Can you work these out from the model? Positions are in its coordinate system, mm. Face numbers are marked on the shaded views. A direction names the side the tool comes from. Round coordinates to 2 decimals unless told otherwise and drop trailing zeros. Write each loop counter-clockwise with the first axis right and the second up, starting at its lowest first coordinate (ties: lowest second). Pieces come first, ordered by that corner, then holes. Notation, with made-up numbers: M 20.5,9 L 41.5,9 A8 cw 41.5,22 Z; hole C 36.25,7.5 d11. An arc over 180 degrees is marked long. Answer as a JSON object with one key per item and string values. Group by question number.
1) Suppose I cut it at D-D, the plane y = 72. Write out the boundary of the cut face in (x, z).
2) Suppose I cut it at C-C, the plane z = -6.75. Write out the boundary of the cut face in (x, y), and give its area (3 significant figures).
3) I'm going to push flat-ended pins straight in: pin 1 Ø0.9 at (x, z) = (-24, -9) entering from +Y; pin 2 Ø1 at (x, z) = (-26, -3.5) entering from -Y; pin 3 Ø2 at (x, y) = (12.5, 17.5) entering from -Z; pin 4 Ø3 at (y, z) = (13.5, -6) entering from +X. Where does each tip first touch, or does it pass through?
4) Suppose I cut it at B-B, the plane x = -2.5. Write out the boundary of the cut face in (y, z).
5) Please list where these lines run through material, in increasing order: L1, parallel to Y at x = 0, z = -1.65; L2, parallel to Z at x = 11.5, y = 18.5; L3, parallel to Y at x = -23, z = 0.25. Write a range as [from, to].
6) On a 3-axis mill with a long thin cutter (end or side, diameter ignored), from which of +Z, -Z, +X, -X, +Y, -Y can I reach the whole of each face in a straight line? I mean the marked faces 4, 5 and 6. Say none if no direction works.
7) If we mould it in two halves opening along Y, with no side actions, what happens to the marked faces 1, 2 and 3? For each: +Y half, -Y half, draft (parallel to the pull), parting line (faces both ways), or undercut.
8) Suppose I cut it at A-A, the plane y = 29.5. Write out the boundary of the cut face in (x, z), and give its area (3 significant figures).
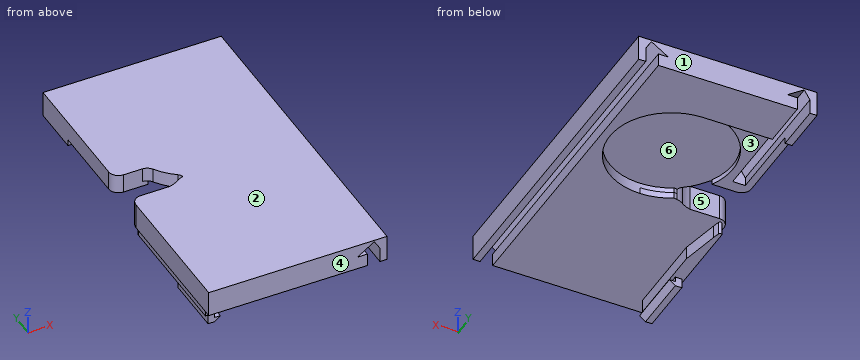
from build123d import *
from build123d.topology import SkipClean

# Parameters (mm, degrees)
SKETCH1_W           = 55
SKETCH1_H           = 8
BOSS_EXTRUDE1_DEPTH = 100
SKETCH4_R           = 19
CUT_EXTRUDE3_DEPTH  = 3.56
CUT_EXTRUDE4_DEPTH  = 2
CUT_EXTRUDE5_DEPTH  = 16
BOSS_EXTRUDE2_START = 2
BOSS_EXTRUDE2_DEPTH = 2
FILLET1_R           = 3
FILLET2_R           = 3
FILLET3_R           = 3
FILLET4_R           = 2
BOSS_EXTRUDE3_DEPTH = 4
CUT_EXTRUDE9_DEPTH  = 39
CUT_EXTRUDE13_DEPTH = 108
BOSS_EXTRUDE4_DEPTH = 18
FILLET5_R           = 0.5


with BuildPart() as part:
    # Sketch1 → Boss-Extrude1 (new body)
    with BuildSketch(Plane(origin=(0, 0, 0), x_dir=(1, 0, 0), z_dir=(0, 1, 0))):
        Rectangle(SKETCH1_W, SKETCH1_H)
    extrude(amount=BOSS_EXTRUDE1_DEPTH)

    # Sketch4 → Cut-Extrude3 (cut)
    with BuildSketch(Plane(origin=(0, 0, -4), x_dir=(-1, 0, 0), z_dir=(0, 0, -1))):
        with Locations((0, 65.948341349)):
            Circle(SKETCH4_R)
    extrude(amount=-CUT_EXTRUDE3_DEPTH, mode=Mode.SUBTRACT)

    # Sketch5 → Cut-Extrude4 (cut)
    with BuildSketch(Plane(origin=(0, 0, -4), x_dir=(-1, 0, 0), z_dir=(0, 0, -1))):
        with BuildLine():
            Line((0, 46.948341349), (27.5, 46.948341349))
            Line((27.5, 46.948341349), (27.5, 84.948341349))
            Line((27.5, 84.948341349), (0, 84.948341349))
            ThreePointArc((0, 84.948341349), (19, 65.948341349), (0, 46.948341349))
        make_face()
    extrude(amount=-CUT_EXTRUDE4_DEPTH, mode=Mode.SUBTRACT)

    # Sketch6 → Cut-Extrude5 (cut)
    with BuildSketch(Plane(origin=(0, 0, -2), x_dir=(-1, 0, 0), z_dir=(0, 0, -1))):
        with BuildLine():
            Line((15.414617012, 46.948341349), (27.5, 46.948341349))
            Line((27.5, 46.948341349), (27.5, 57.34244177))
            Line((27.5, 57.34244177), (16.93925891, 57.34244177))
            ThreePointArc((16.93925891, 57.34244177), (13.716933305, 52.801260277), (9.316482273, 49.389260515))
            add(Edge.make_bspline(
                [(9.316482273, 49.389260515), (9.656060905, 49.327672788), (9.995639536, 49.266085061), (10.335218168, 49.204497334)],
                knots=[0, 0, 0, 0, 0.453327557, 0.453327557, 0.453327557, 0.453327557], degree=3))
            ThreePointArc((10.335218168, 49.204497334), (11.386910009, 48.891383158), (12.344973185, 48.356396089))
            ThreePointArc((12.344973185, 48.356396089), (13.813009587, 47.506772296), (15.414617012, 46.948341349))
        make_face()
    extrude(amount=-CUT_EXTRUDE5_DEPTH, mode=Mode.SUBTRACT)

    # Sketch7 → Boss-Extrude2 (add)
    with BuildSketch(Plane(origin=(0, 0, -2), x_dir=(-1, 0, 0), z_dir=(0, 0, -1)).offset(BOSS_EXTRUDE2_START)):
        with BuildLine():
            Line((0, 46.948341349), (15.414617012, 46.948341349))
            ThreePointArc((15.414617012, 46.948341349), (13.813009587, 47.506772296), (12.344973185, 48.356396089))
            ThreePointArc((12.344973185, 48.356396089), (11.386910009, 48.891383158), (10.335218168, 49.204497334))
            Line((10.335218168, 49.204497334), (9.316482273, 49.389260515))
            ThreePointArc((9.316482273, 49.389260515), (4.815468002, 47.568698591), (0, 46.948341349))
        make_face()
    extrude(amount=-BOSS_EXTRUDE2_DEPTH)

    # Fillet1
    fillet1_edges = [part.edges().sort_by_distance(p)[0] for p in [
        (-27.5, 46.948341349, 0),
    ]]
    fillet(fillet1_edges, radius=FILLET1_R)

    # Fillet2
    fillet2_edges = [part.edges().sort_by_distance(p)[0] for p in [
        (-27.5, 57.34244177, 1),
    ]]
    fillet(fillet2_edges, radius=FILLET2_R)

    # Fillet3
    fillet3_edges = [part.edges().sort_by_distance(p)[0] for p in [
        (-16.93925891, 57.34244177, 1.78),
    ]]
    fillet(fillet3_edges, radius=FILLET3_R)

    # Fillet4
    # the kernel refuses this fillet: 2 mm, written as the material it adds along each edge
    with BuildSketch(Plane(origin=(-9.316482273, 49.389260515, -0.44), x_dir=(-0.8420947177301665, 0.5393296639078471, 0), z_dir=(0, 0, 1))) as fillet4_piece_1:
        with BuildLine():
            CenterArc((2.285143138, 1.996733658), FILLET4_R, 220.22985095, 46.495139538)
            Line((0.758223851, 0.705022587), (0, 0))
            ThreePointArc((0, 0), (1.08544299, 0.031030246), (2.170885981, 0))
        make_face()
    extrude(amount=4.44)

    # Sketch8 → Boss-Extrude3 (add)
    with SkipClean():  # the faces are left unmerged after this step: merging them gives an invalid solid
        with BuildSketch(Plane(origin=(0, 0, -4), x_dir=(-1, 0, 0), z_dir=(0, 0, -1))):
            with BuildLine():
                Line((26.088640722, 4.806504153), (22.273821869, 4.806504153))
                Line((22.273821869, 4.806504153), (22.273821869, 31.413664101))
                Line((22.273821869, 31.413664101), (24.599018881, 43.221316386))
                ThreePointArc((24.599018881, 43.221316386), (25.224862201, 45.756953754), (26.088640722, 48.221710007))
                Line((26.088640722, 48.221710007), (26.088640722, 4.806504153))
            make_face()
        extrude(amount=BOSS_EXTRUDE3_DEPTH)

    # Sketch10 → Cut-Extrude9 (cut)
    with SkipClean():  # the faces are left unmerged after this step: merging them gives an invalid solid
        with BuildSketch(Plane(origin=(0, 100, 0), x_dir=(1, 0, 0), z_dir=(0, 1, 0))):
            Polygon((-21.421951451, 4), (-25.321951451, 4), (-25.321951451, -0.657162479), (-23.589826686, -3.532235176), (-18.397407116, 0), (-21.421951451, 0), align=None)
        extrude(amount=-CUT_EXTRUDE9_DEPTH, mode=Mode.SUBTRACT)

    # Sketch11 → Cut-Extrude13 (cut)
    with SkipClean():  # the faces are left unmerged after this step: merging them gives an invalid solid
        with BuildSketch(Plane(origin=(0, 100, 0), x_dir=(1, 0, 0), z_dir=(0, 1, 0))):
            Polygon((21.421951451, 4), (25.321951451, 4), (25.321951451, -0.657162479), (23.589826686, -3.532235176), (18.397407116, 0), (21.421951451, 0), align=None)
        extrude(amount=-CUT_EXTRUDE13_DEPTH, mode=Mode.SUBTRACT)

    # Sketch12 → Boss-Extrude4 (add)
    with SkipClean():  # the faces are left unmerged after this step: merging them gives an invalid solid
        with BuildSketch(Plane.XZ.offset(-4.806504153)):
            Polygon((-23.25622165, -11.019758414), (-21.45622165, -9.537592081), (-23.25622165, -9.537592081), (-23.25622165, -8), (-25.25622165, -8), (-25.25622165, -9.537592081), (-25.25622165, -11.019758414), align=None)
        extrude(amount=-BOSS_EXTRUDE4_DEPTH)

    # Fillet5
    # the kernel refuses this fillet: 0.5 mm, written as the material it takes off along each edge
    with BuildSketch(Plane(origin=(-26.088640722, 48.221710007, -4), x_dir=(0, -1, 0), z_dir=(0, 0, -1))) as fillet5_piece_1:
        with BuildLine():
            CenterArc((3.006099278, -0.5), FILLET5_R, 90, 164.292569468)
            ThreePointArc((2.870736632, -0.981328322), (1.421812921, -0.530318544), (0, 0))
            Line((0, 0), (3.006099278, 0))
        make_face()
    extrude(amount=11.584578962, mode=Mode.SUBTRACT)


solid = part.part
Results:
{
 "1": {"outline": "M -27.5,-2 L -25.32,-2 L -25.32,0.66 L -23.59,3.53 L -18.4,0 L -21.42,0 L -21.42,-2 L -18.01,-2 L -18.01,-0.44 L 18.01,-0.44 L 18.01,-4 L 21.42,-4 L 21.42,0 L 18.4,0 L 23.59,3.53 L 25.32,0.66 L 25.32,-4 L 27.5,-4 L 27.5,4 L -27.5,4 Z"},
 "2": {"outline": "M -26.09,4.81 L -22.27,4.81 L -22.27,31.41 L -24.6,43.22 A27.47 ccw -25.11,45.35 A0.5 ccw -26.09,45.22 Z", "area": "136 mm^2"},
 "3": {"pin 1": "y = 22.81", "pin 2": "y = 0", "pin 3": "z = -4", "pin 4": "x = -22.27"},
 "4": {"outline": "M 0,-4 L 47.11,-4 L 47.11,-0.44 L 84.78,-0.44 L 84.78,-2 L 84.95,-2 L 84.95,-4 L 100,-4 L 100,4 L 0,4 Z"},
 "5": {"L1": "[0, 46.95], [84.95, 100]", "L2": "[-4, 4]", "L3": "[0, 46.95], [57.34, 61]"},
 "6": {"face 4": "+Z, -Z, +X, -X, -Y", "face 5": "+Z, -Z, -X", "face 6": "-Z"},
 "7": {"face 1": "+Y half", "face 2": "draft", "face 3": "undercut"},
 "8": {"outline": "M -27.5,-4 L -26.09,-4 L -26.09,-8 L -22.27,-8 L -22.27,-4 L 21.42,-4 L 21.42,0 L 18.4,0 L 23.59,3.53 L 25.32,0.66 L 25.32,-4 L 27.5,-4 L 27.5,4 L -27.5,4 Z", "area": "427 mm^2"}
}
